Design review of the part built by this model. Coordinates are the model's own, in mm. Face numbers are marked on the shaded views. A direction names the side the tool comes from. Coordinates: 2 decimals unless noted, no trailing zeros. Write each loop counter-clockwise with the first axis right and the second up, starting at its lowest first coordinate (ties: lowest second). Pieces come first, ordered by that corner, then holes. Notation, with made-up numbers: (-28, 1) -> (14, 1) arc R15 cw to (14, 26) -> close; hole circle Ø2 at (35.25, -12). An arc over 180 degrees is marked (long way). Return JSON: item names as keys, results as strings. Group by question number.
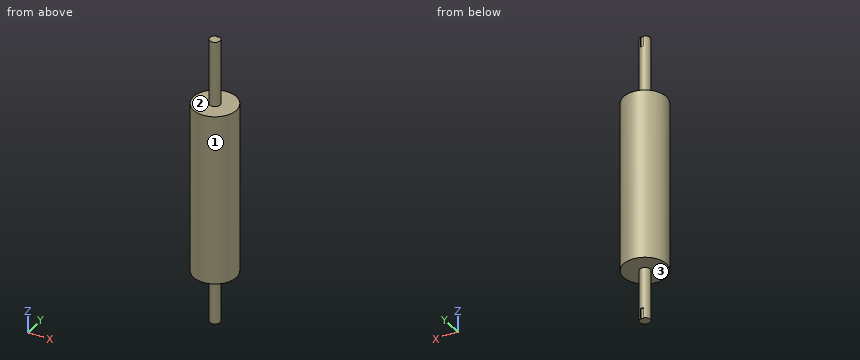
from build123d import *

# Parameters (mm, degrees)
SKETCH2_R           = 125
BOSS_EXTRUDE1_DEPTH = 1000
SKETCH7_R           = 30
BOSS_EXTRUDE3_DEPTH = 384.03
BOSS_EXTRUDE4_START = 300
SKETCH8_R           = 30
BOSS_EXTRUDE4_DEPTH = 300
SKETCH18_W          = 18
SKETCH18_H          = 11
CUT_EXTRUDE2_DEPTH  = 60
SKETCH19_W          = 18
SKETCH19_H          = 11
CUT_EXTRUDE3_DEPTH  = 60


with BuildPart() as part:
    # Sketch2 → Boss-Extrude1 (new body)
    with BuildSketch(Plane.XY):
        Circle(SKETCH2_R)
    extrude(amount=BOSS_EXTRUDE1_DEPTH)

    # Sketch7 → Boss-Extrude3 (add)
    with BuildSketch(Plane.XY.offset(1000)):
        Circle(SKETCH7_R)
    extrude(amount=BOSS_EXTRUDE3_DEPTH)

    # Sketch8 → Boss-Extrude4 (add)
    with BuildSketch(Plane(origin=(0, 0, 0), x_dir=(-1, 0, 0), z_dir=(0, 0, -1)).offset(BOSS_EXTRUDE4_START)):
        with Locations(Location((0, 0, 0), (0, 0, 180))):
            Circle(SKETCH8_R)
    extrude(amount=-BOSS_EXTRUDE4_DEPTH)

    # Sketch18 → Cut-Extrude2 (cut)
    with BuildSketch(Plane.XY.offset(1384.03)):
        with Locations((0, 30)):
            Rectangle(SKETCH18_W, SKETCH18_H)
    extrude(amount=-CUT_EXTRUDE2_DEPTH, mode=Mode.SUBTRACT)

    # Sketch19 → Cut-Extrude3 (cut)
    with BuildSketch(Plane(origin=(0, 0, -300), x_dir=(-1, 0, 0), z_dir=(0, 0, -1))):
        with Locations((0, 30)):
            Rectangle(SKETCH19_W, SKETCH19_H)
    extrude(amount=-CUT_EXTRUDE3_DEPTH, mode=Mode.SUBTRACT)


solid = part.part
Q1. Wall thickness on L1, parallel to Z at x = -93.5, y = -3; L2, parallel to Y at x = 0, z = 618.5; L3, parallel to X at y = 89, z = 998: over which ranges is each line inside the solid? List them lowest first.
Q2. We need section C-C on y = 68.5. Write out the cut boundary in (x, z).
Q3. We need section A-A on y = 0. Write out the cut boundary in (x, z), plus the area to 3 significant figures.
Q4. For the marked faces 1, 2 and 3, list the 3-axis set-ups (+Z, -Z, +X, -X, +Y, -Y) from which the entire face can be reached by the end or side of a thin tool; tool diameter is ignored.
Q5. For P1, Ø1.6, axis at x = 1, y = 27.5, coming from the +Z side; P2, Ø9, axis at x = -3, z = 1342.5, coming from the +Y side; P3, Ø1.2, axis at y = 27, z = 1357.5, coming from the -X side, all flat-tipped, find the tip position at first contact; note any pin that passes through.
Q6. We need section D-D on y = -80. Write out the cut boundary in (x, z), plus the area to 3 significant figures.
Q7. We need section B-B on z = -26.5. Write out the cut boundary in (x, y).
Findings below:
{
 "1": {"L1": "z = 0 to 1000", "L2": "y = -125 to 125", "L3": "x = -87.77 to 87.77"},
 "2": {"outline": "(-104.56, 0) -> (104.56, 0) -> (104.56, 1000) -> (-104.56, 1000) -> close"},
 "3": {"outline": "(-125, 0) -> (-30, 0) -> (-30, -300) -> (30, -300) -> (30, 0) -> (125, 0) -> (125, 1000) -> (30, 1000) -> (30, 1384.03) -> (-30, 1384.03) -> (-30, 1000) -> (-125, 1000) -> close", "area": "291,000 mm^2"},
 "4": {"face 1": "+Z, -Z", "face 2": "+Z", "face 3": "-Z"},
 "5": {"P1": "stops at z = 1324.03", "P2": "stops at y = 24.5", "P3": "stops at x = -14.25"},
 "6": {"outline": "(-96.05, 0) -> (96.05, 0) -> (96.05, 1000) -> (-96.05, 1000) -> close", "area": "192,000 mm^2"},
 "7": {"outline": "circle Ø60 at (0, 0)"}
}
